Autodesk Inventor part; units mm, degrees
ref_plane "Work Plane1" through (18.5742, 0, 0) normal (0, 0, -1) x (1, 0, 0)
ref_plane "YZ Plane" through (0, 0, 0) normal (1, 0, 0) x (0, 1, 0)
ref_plane "XZ Plane" through (0, 0, 0) normal (0, 1, 0) x (-1, 0, 0)
sketch "Szkic1" plane through (0, 0, 0) normal (0, 0, 1) x (1, 0, 0)
  line L0 (0, 0) -> (3, 0)
  line L1 (0, 0) -> (0, 2.5)
  line L2 (3, 2) -> (3, 0)
  line L3 (0, 2.5) -> (3.5265, 7.0347)
  line L4 (3, 2) -> (6.3108, 3.1351)
  arc A0 (6.3108, 3.1351) -> (3.5265, 7.0347) centre (5.5, 5.5) ccw
  line L5 (3, 2) -> (0, 2.5)
  line L6 (3, 2) -> (0, 0.9714)
  dimension "d0" = 4
  dimension "d1" = 5.5
  dimension "d2" = 5.5
  dimension "d3" = 2.5
  dimension "d4" = 3
  dimension "d5" = 5
revolve "Bryła" add sketch "Szkic1" angle 360 about axis through (0, 0, 0) along (1, 0, 0) contours L1 L6 L2 L0 | L1 L5 L6
extrude "Skrzydło1" add sketch "Szkic1" along normal mid plane 2.5 contours L1 L5 L6 | L5 L3 A0 L4
fillet "Zaokrąglenie1" [suppressed]
mirror "Skrzydło2" about plane through (0, 0, 0) normal (0, 1, 0) of "Skrzydło1"
sketch "Szkic2" plane through (0, 0, 0) normal (1, 0, 0) x (0, 1, 0)
  line L0 (0, -14) -> (0, 14)
  line L1 (-14, 0) -> (14, 0)
  point P0 (0, 0)
hole "Gwint" at (0, 0, 0) direction (1, 0, 0) diameter 2.459 end through all
chamfer "Faza1" distance 0.2706 angle 30 1 edges at (0, 0, -1.2295) measured on face at (0, -2.0735, 0.0494)
ref_plane "Work Plane1" through (18.5742, 0, 0) normal (0, 0, -1) x (1, 0, 0)
equation "\"d0\" = KOD2"
equation "\"d1\" = KOH1 - RR"
equation "\"d2\" = 0.5 * E0 - RR"
equation "\"d3\" = RR"
equation "\"d4\" = KOH"
equation "\"d5\" = KOD"
equation "\"d6\" = SW"
equation "\"d8\" = 0.333333 * SW"
equation "\"d9\" = -0.5 * GD1 + 0.5 * NND"
equation "\"d109\" = -0.5 * GD1 + 0.5 * NND"
equation "\"NND\" = 3"
equation "\"KOH\" = 3"
equation "\"KOH1\" = 8"
equation "\"SW\" = 2.5"
equation "\"KOD\" = 5"
equation "\"KOD2\" = 4"
equation "\"RR\" = 2.5"
equation "\"E0\" = 16"
equation "\"GUL\" = 0.541266 * PTC"
equation "\"PTC\" = 0.5"
equation "\"THREADDIA\" = 3"
equation "\"TOA\" = 30deg"
equation "\"RR2\" = 1.6"
equation "\"SW1\" = 3"
equation "\"GAL\" = 0.541266 * PTC"
properties part number "KS B 1014 - M 3" material "Stal, miękka"
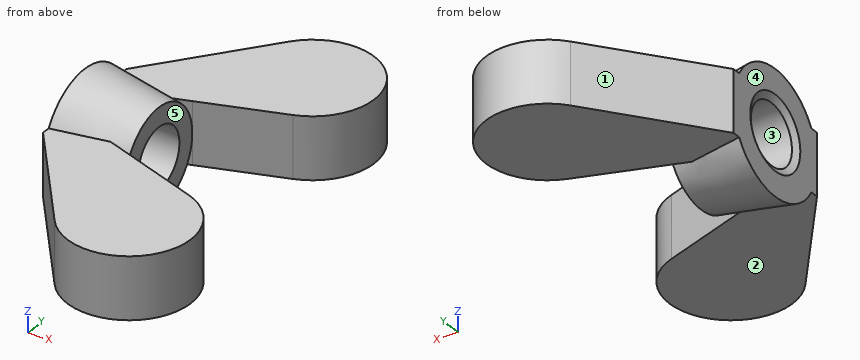
Geometry: final body of the model. Coordinates: model frame, mm. Face numbers are marked on the shaded views. A direction names the side the tool comes from. Give positions to 0.01 mm unless a question says otherwise; leave off trailing zeros. Write each loop counter-clockwise with the first axis right and the second up, starting at its lowest first coordinate (ties: lowest second). Pieces come first, ordered by that corner, then holes.
1. Draft query along Z for the marked faces 1, 2 and 3. Return one class per face: released by +Z, released by -Z, zero draft, split by the parting line, or undercut.
2. Section query B-B, the plane x = 3.75. Return loops of the section in (y, z), then the cut area to 3 significant figures.
3. Reachability of the marked faces 4 and 5 from +Z, -Z, +X, -X, +Y, -Y: full face, straight path, thin tool, end or side. Return the list, or none.
4. Section query A-A, the plane y = 0. Return loops of the section in (x, z), then the cut area to 3 significant figures.
5. Line query: probe 1 along Y at (x, z) = (6.25, -0.8); probe 2 along Z at (x, y) = (0.95, 0); probe 3 along Z at (x, y) = (5.5, 6.25). Output: solid intervals per line, ascending.
6. Pin query (flat end, axial travel): P1, Ø3, axis at x = 2, y = 5, coming from the -Z side; P2, Ø2, axis at x = 6.5, y = 1.5, coming from the -Z side; P3, Ø3, axis at x = 5.5, y = -4.5, coming from the +Z side; P4, Ø4, axis at x = 4.5, y = 0, coming from the -Z side. Return the tip coordinate at first contact, or that it passes through.
7. Section query D-D, the plane y = 6. Return loops of the section in (x, z), then the cut area to 3 significant figures.
8. Section query C-C, the plane x = 2.75. Return loops of the section in (y, z), then the cut area to 3 significant figures.
Computed:
1. face 1: zero draft
1. face 2: released by -Z
1. face 3: undercut
2. outline: (-7.29, -1.25) - (-2.26, -1.25) - (-2.26, 1.25) - (-7.29, 1.25) - close; (2.26, -1.25) - (7.29, -1.25) - (7.29, 1.25) - (2.26, 1.25) - close
2. area: 25.1 mm2
3. face 4: +Z, -Z, -X, +Y, -Y
3. face 5: +Z, -Z, +X
4. outline: (0, -2.5) - (3, -2) - (3, -1.23) - (0.16, -1.23) - (0, -1.5) - close; (0, 1.5) - (0.16, 1.23) - (3, 1.23) - (3, 2) - (0, 2.5) - close
4. area: 6.08 mm2
5. probe 1: y = -7.88 to -3.11, 3.11 to 7.88
5. probe 2: z = -2.34 to -1.23, 1.23 to 2.34
5. probe 3: z = -1.25 to 1.25
6. P1: stops at z = -1.25
6. P2: passes through
6. P3: stops at z = 1.25
6. P4: stops at z = -2.08
7. outline: (2.72, -1.25) - (7.95, -1.25) - (7.95, 1.25) - (2.72, 1.25) - close
7. area: 13.1 mm2
8. outline: (-6.04, -1.25) - (-1.91, -1.25) - (-1.91, -0.71) arc R2.04 ccw to (1.91, -0.71) - (1.91, -1.25) - (6.04, -1.25) - (6.04, 1.25) - (1.91, 1.25) - (1.91, 0.71) arc R2.04 ccw to (-1.91, 0.71) - (-1.91, 1.25) - (-6.04, 1.25) - close; hole circle Ø2.46 at (0, 0)
8. area: 28.7 mm2
